For this review, take the finished solid that the model builds, in its own axes (mm). Round coordinates to 2 decimals unless told otherwise and drop trailing zeros. Write each loop counter-clockwise with the first axis right and the second up, starting at its lowest first coordinate (ties: lowest second). Pieces come first, ordered by that corner, then holes.
Autodesk Inventor part; units mm, degrees
ref_plane "YZ Plane" through (0, 0, 0) normal (1, 0, 0) x (0, 1, 0)
ref_plane "XZ Plane" through (0, 0, 0) normal (0, 1, 0) x (-1, 0, 0)
ref_plane "XY Plane" through (0, 0, 0) normal (0, 0, 1) x (1, 0, 0)
sketch "Sketch1" plane through (0, 0, 0) normal (0, 1, 0) x (-1, 0, 0)
  circle A0 centre (0, 0) radius 99.695
  circle A1 centre (0, 0) radius 34.925
  dimension "d0" = 199.39
  dimension "d16" = 69.85
extrude "Extrusion1" add sketch "Sketch1" along normal blind 2.54
sketch "Sketch2" plane through (0, 2.54, 0) normal (0, 1, 0) x (1, 0, 0)
  line L0 (0, 0) -> (33.676, 33.676) construction
  line L1 (0, 0) -> (47.625, 0) construction
  dimension "d4" = 47.625
  dimension "d5" = 45
hole "Hole1" at (33.676, 2.54, -33.676) direction (0, -1, 0) diameter 2.8448 end through all
pattern_circular "Circular Pattern1" count 6 over 360 about axis through (0, 0, 0) along (0, 1, 0) of "Hole1"
properties part number "4K shield bottom" material "Brass, Soft Yellow"
(1) We need section A-A, the plane x = 0. Give the boundary of the cut face in (y, z) (3 decimals).
Geometry check:
outline: (0, -99.695) - (2.54, -99.695) - (2.54, -34.925) - (0, -34.925) - close; (0, 34.925) - (2.54, 34.925) - (2.54, 99.695) - (0, 99.695) - close
(2) We need section C-C, the plane y = 1.3. Give the boundary of the cut face in (x, z) (3 decimals).
Geometry check:
outline: circle Ø199.39 at (0, 0); hole circle Ø2.845 at (-46.002, -12.326); hole circle Ø2.845 at (-33.676, 33.676); hole circle Ø69.85 at (0, 0); hole circle Ø2.845 at (-12.326, -46.002); hole circle Ø2.845 at (12.326, 46.002); hole circle Ø2.845 at (33.676, -33.676); hole circle Ø2.845 at (46.002, 12.326)
(3) Mouldability with a two-part tool opening along X and no side actions: class faces 1 (the face through (-43, 2.54, 1)), 2 (the face through (21.612, 1.252, 97.324)), 3 (the face through (27.715, 1.252, 21.251)) as pulls with the +X half, pulls with the -X half, needs draft (parallel to the pull), parting line crosses it, or undercut.
Geometry check:
face 1: needs draft
face 2: parting line crosses it
face 3: undercut
(4) We need section B-B, the plane z = 0. Give the boundary of the cut face in (x, y) (3 decimals).
Geometry check:
outline: (-99.695, 0) - (-34.925, 0) - (-34.925, 2.54) - (-99.695, 2.54) - close; (34.925, 0) - (99.695, 0) - (99.695, 2.54) - (34.925, 2.54) - close
(5) We need section D-D, the plane x = -70.5. Give the boundary of the cut face in (y, z), and give its area (3 significant figures).
Geometry check:
outline: (0, -70.49) - (2.54, -70.49) - (2.54, 70.49) - (0, 70.49) - close
area: 358 mm2
(6) For pin 1 Ø1 at (x, z) = (-31, -73) entering from -Y; pin 2 Ø2.5 at (x, z) = (-46, -12.33) entering from -Y, all flat-tipped, find the tip position at first contact; note any pin that passes through.
Geometry check:
pin 1: stops at y = 0
pin 2: passes through
(7) For line 1 along Z through (x, y) = (13.5, 2.1); line 2 along Z through (x, y) = (0, 1.35) (3 decimals); line 3 along X through (y, z) = (1.35, 2), list the stretches that pass through material, from the lowest coordinate up.
Geometry check:
line 1: z = -98.78 to -32.21, 32.21 to 45.2, 46.81 to 98.78
line 2: z = -99.695 to -34.925, 34.925 to 99.695
line 3: x = -99.67 to -34.87, 34.87 to 99.67
